Build history of the part. All positions in model axes, mm. Face numbers are marked on the shaded views. Give positions to 0.01 mm unless a question says otherwise; leave off trailing zeros. Loops run counter-clockwise (first coordinate to the right, second up) from the corner with the lowest first, then second, coordinate; pieces in that order, holes last. Notation, with made-up numbers: M 35.25,36 L 56.25,36 A34 cw 56.25,68 Z; hole C 33,-2.5 d7. An arc over 180 degrees is marked long. Put each result on its own line as item: value.
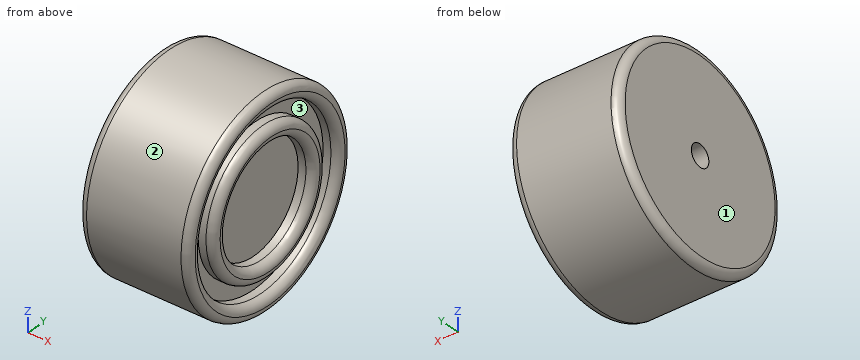
```python
from build123d import *

# Parameters (mm, degrees)
F0_W     = 2
F0_H     = 2
F0_W_2   = 12
F2_R     = 0.99999
F3_R     = 1.4
F4_DEPTH = 10


# Not quite as in the source:
# - a fillet or chamfer is up to 0.001 mm smaller than in the source, because OpenCascade refuses the exact size


with BuildPart() as f1:
    # F0 (on Front) → F1 (revolve)
    with BuildSketch(Plane.XZ):
        Polygon((-12, 0), (0, 0), (0, 7), (0, 9), (0, 11), (-12, 11), align=None)
        with Locations((1, 8)):
            Rectangle(F0_W, F0_H)
        with Locations((-6, 12)):
            Rectangle(F0_W_2, F0_H)
        with Locations((1, 12)):
            Rectangle(F0_W, F0_H)
    revolve(axis=Axis((-6, 0, 0), (-1, 0, 0)))

    # F2 (radius 1 in the source; OpenCascade refuses exactly that, so slightly less here)
    f2_edges = [f1.edges().sort_by_distance(p)[0] for p in [
        (2, 0, -13),
        (2, 0, -9),
        (2, 0, -7),
        (2, 0, -11),
        (-12, 0, -13),
    ]]
    fillet(f2_edges, radius=F2_R)

    # F3 (on face) → F4 (cut)
    with BuildSketch(Plane(origin=(-12, 0, 0), x_dir=(0, -1, 0), z_dir=(-1, 0, 0))):
        Circle(F3_R)
    extrude(amount=-F4_DEPTH, mode=Mode.SUBTRACT)


solid = f1.part
```
Q1. Probe line 1 (Y direction, x = 0.5, z = 0); line 2 (X direction, y = 2.5, z = -10.25); line 3 (Z direction, x = 0.75, y = -2). List the from-to ranges inside material, lowest first. Write a range as from..to.
Here are the results:
line 1: -13..-11, -9..-7, 7..9, 11..13
line 2: -12..0
line 3: -12.85..-10.82, -8.77..-6.71, 6.71..8.77, 10.82..12.85
Q2. Drop flat-ended pins along their axis: pin 1 Ø6 at (x, y) = (-1, -9) entering from -Z; pin 2 Ø1.5 at (x, y) = (-2, -3.5) entering from +Z; pin 3 Ø6 at (x, z) = (-3.5, -8) entering from -Y. Give the stop position or say it passes through.
Here are the results:
pin 1: z = -11.53
pin 2: z = 12.71
pin 3: y = -12
Q3. Mould opens along Y. For the marked faces 1, 2 and 3 say: pulls with the +Y half, pulls with the -Y half, needs draft (parallel to the pull), parting line crosses it, or undercut.
Here are the results:
face 1: needs draft
face 2: parting line crosses it
face 3: undercut
Q4. Slice it at B-B (x = -10.5). List the corners of the cut face in (y, z).
Here are the results:
outline: C 0,0 d26; hole C 0,0 d2.8
